```python
from build123d import *

# Parameters (mm, degrees)
F0_W     = 45
F0_H     = 3.5
F1_DEPTH = 75
F2_R     = 5
F3_DEPTH = 3.5
F4_R     = 1


with BuildPart() as f1:
    # F0 (on Front) → F1 (new body, symmetric)
    with BuildSketch(Plane.XZ):
        with Locations((22.5, 1.75)):
            Rectangle(F0_W, F0_H)
    extrude(amount=F1_DEPTH, both=True)

    # F2 (on Top) → F3 (cut, through all)
    with BuildSketch(Plane.XY):
        with Locations((14, 0)):
            Circle(F2_R)
    extrude(amount=F3_DEPTH, mode=Mode.SUBTRACT)

    # F4
    f4_edges = [f1.edges().sort_by_distance(p)[0] for p in [
        (0, 0, 3.5),
        (0, 0, 0),
    ]]
    fillet(f4_edges, radius=F4_R)


solid = f1.part
```
Verification items for the finished model (mm, model axes). Round coordinates to 2 decimals unless told otherwise and drop trailing zeros. Write each loop counter-clockwise with the first axis right and the second up, starting at its lowest first coordinate (ties: lowest second). Pieces come first, ordered by that corner, then holes. Notation, with made-up numbers: (-10, -29) - (3, -29) arc R28 cw to (3, 0) - close; hole circle Ø8 at (49, -25.75). An arc over 180 degrees is marked (long way). Answer as a JSON object with one key per item and string values. Group by question number.
Q1. Mould release check, pull along X, two halves, no side actions. Record for faces 1 (the flat face through (45, -1, 2)), 2 (the flat face through (23, -1, 3.5)), 3 (the cylindrical face through (18.77, 1.5, 1.73)): released by +X, released by -X, zero draft, split by the parting line, or undercut.
Q2. Section check B-B, the plane y = 0. Enter the section's corners in (x, z), plus the area to 3 significant figures.
Q3. Thickness scan on line 1 (Y direction, x = 14, z = 1.35); line 2 (X direction, y = -19.5, z = 2.55); line 3 (Y direction, x = 17.5, z = 0.75). Record the ranges inside material, lowest first.
Q4. Section check A-A, the plane x = 14. Enter the section's corners in (y, z), plus the area to 3 significant figures.
Found:
{
 "1": {"face 1": "released by +X", "face 2": "zero draft", "face 3": "undercut"},
 "2": {"outline": "(0, 1) arc R1 ccw to (1, 0) - (9, 0) - (9, 3.5) - (1, 3.5) arc R1 ccw to (0, 2.5) - close; (19, 0) - (45, 0) - (45, 3.5) - (19, 3.5) - close", "area": "122 mm^2"},
 "3": {"line 1": "y = -75 to -5, 5 to 75", "line 2": "x = 0 to 45", "line 3": "y = -75 to -3.57, 3.57 to 75"},
 "4": {"outline": "(-75, 0) - (-5, 0) - (-5, 3.5) - (-75, 3.5) - close; (5, 0) - (75, 0) - (75, 3.5) - (5, 3.5) - close", "area": "490 mm^2"}
}
